from build123d import *

# Parameters (mm, degrees)
F0_W     = 1117.6
F0_H     = 889
F1_DEPTH = 50.8
F0_W_2   = 1219.2
F0_H_2   = 990.6
F2_DEPTH = 12.7
F3_R     = 3.175


with BuildPart() as f1:
    # F0 (on Front) → F1 (new body)
    with BuildSketch(Plane.XZ):
        with BuildLine():
            Line((-565.15, -457.2), (565.15, -457.2))
            ThreePointArc((565.15, -457.2), (569.640128, -455.340128), (571.5, -450.85))
            Line((571.5, -450.85), (571.5, 450.85))
            ThreePointArc((571.5, 450.85), (569.640128, 455.340128), (565.15, 457.2))
            Line((565.15, 457.2), (-565.15, 457.2))
            ThreePointArc((-565.15, 457.2), (-569.640128, 455.340128), (-571.5, 450.85))
            Line((-571.5, 450.85), (-571.5, -450.85))
            ThreePointArc((-571.5, -450.85), (-569.640128, -455.340128), (-565.15, -457.2))
        make_face()
        Rectangle(F0_W, F0_H, mode=Mode.SUBTRACT)
    extrude(amount=F1_DEPTH)

    # F0 (on Front) → F2 (join)
    with BuildSketch(Plane.XZ):
        Rectangle(F0_W_2, F0_H_2)
        with BuildLine():
            ThreePointArc((571.5, -450.85), (569.640128, -455.340128), (565.15, -457.2))
            Line((565.15, -457.2), (-565.15, -457.2))
            ThreePointArc((-565.15, -457.2), (-569.640128, -455.340128), (-571.5, -450.85))
            Line((-571.5, -450.85), (-571.5, 450.85))
            ThreePointArc((-571.5, 450.85), (-569.640128, 455.340128), (-565.15, 457.2))
            Line((-565.15, 457.2), (565.15, 457.2))
            ThreePointArc((565.15, 457.2), (569.640128, 455.340128), (571.5, 450.85))
            Line((571.5, 450.85), (571.5, -450.85))
        make_face(mode=Mode.SUBTRACT)
    extrude(amount=F2_DEPTH)

    # F3
    f3_edges = [f1.edges().sort_by_distance(p)[0] for p in [
        (-609.6, -12.7, 0),
        (609.6, -12.7, 0),
    ]]
    fillet(f3_edges, radius=F3_R)


solid = f1.part
Model file for the job. Use its own axes, mm. A direction names the side the tool comes from. Coordinates: 2 decimals unless noted, no trailing zeros. Write each loop counter-clockwise with the first axis right and the second up, starting at its lowest first coordinate (ties: lowest second). Pieces come first, ordered by that corner, then holes. Notation, with made-up numbers: (71.5, 62) -> (89.5, 62) arc R13 ccw to (89.5, 74) -> close; hole circle Ø4 at (80.25, 20.25). An arc over 180 degrees is marked (long way). One line per item, written item: value. Start each with the question number.
1) Slice it at A-A on z = 225. Write the cut outline in (x, y) (3 decimals), then the cut area to 3 significant figures.
2) Which spindle directions (+Z, -Z, +X, -X, +Y, -Y) get a long thin tool onto all of the face, cutting with end or side? Do faces 1 (the face through (-8, -25, 444.5)), 2 (the face through (8, -31, 457.2)), 3 (the face through (-48, -12.7, -475)). Say none if no direction does.
3) Probe probe 1 along X at (y, z) = (-38.5, -251.5); probe 2 along Z at (x, y) = (-523, -16.5); probe 3 along Z at (x, y) = (489, -5). List the from-to ranges inside material, lowest first.
4) Flat gauge pins, fed straight in: pin 1 Ø6 at (y, z) = (-42, -285.5) entering from +X; pin 2 Ø10 at (y, z) = (-39, -173.5) entering from -X; pin 3 Ø10 at (x, y) = (-172, -35) entering from -Z. Where does each tip first touch, or does it go through?
5) Slice it at B-B on x = 144. Write the cut outline in (y, z), then the cut area to 3 significant figures.
6) Pull direction X, two halves, no side cores. Call faces 4 (the face through (-48, 0, -475)), 5 (the face through (-571.5, -31, 6)), 6 (the face through (558.8, -25, -6)): +X half, -X half, draft (parallel to the pull), parting line (faces both ways), or undercut.
7) Slice it at C-C on y = -27. Write the cut outline in (x, z), then the cut area to 3 significant figures.
Answers follow:
1. outline: (-609.6, -9.525) arc R3.175 ccw to (-606.425, -12.7) -> (-571.5, -12.7) -> (-571.5, -50.8) -> (-558.8, -50.8) -> (-558.8, 0) -> (-609.6, 0) -> close; (558.8, -50.8) -> (571.5, -50.8) -> (571.5, -12.7) -> (606.425, -12.7) arc R3.175 ccw to (609.6, -9.525) -> (609.6, 0) -> (558.8, 0) -> close
1. area: 2,250 mm2
2. face 1: +Y, -Y
2. face 2: +Z, +X, -X, -Y
2. face 3: -Y
3. probe 1: -571.5 to -558.8, 558.8 to 571.5
3. probe 2: -457.2 to -444.5, 444.5 to 457.2
3. probe 3: -495.3 to -444.5, 444.5 to 495.3
4. pin 1: x = 571.5
4. pin 2: x = -571.5
4. pin 3: z = -457.2
5. outline: (-50.8, -457.2) -> (-12.7, -457.2) -> (-12.7, -495.3) -> (0, -495.3) -> (0, -444.5) -> (-50.8, -444.5) -> close; (-50.8, 444.5) -> (0, 444.5) -> (0, 495.3) -> (-12.7, 495.3) -> (-12.7, 457.2) -> (-50.8, 457.2) -> close
5. area: 2,260 mm2
6. face 4: draft
6. face 5: -X half
6. face 6: undercut
7. outline: (-571.5, -450.85) arc R6.35 ccw to (-565.15, -457.2) -> (565.15, -457.2) arc R6.35 ccw to (571.5, -450.85) -> (571.5, 450.85) arc R6.35 ccw to (565.15, 457.2) -> (-565.15, 457.2) arc R6.35 ccw to (-571.5, 450.85) -> close; hole (-558.8, -444.5) -> (558.8, -444.5) -> (558.8, 444.5) -> (-558.8, 444.5) -> close
7. area: 51,600 mm2
